```python
from build123d import *

# Parameters (mm, degrees)
EXTRUDE_1_DEPTH     = 10
CUT_EXTRUDE_1_DEPTH = 140.112364655
SKETCH_3_W          = 30
SKETCH_3_H          = 10
SKETCH_3_W_2        = 75
SKETCH_3_H_2        = 20
CUT_EXTRUDE_2_DEPTH = 140.112364655
SKETCH_4_W          = 25
SKETCH_4_H          = 10
EXTRUDE_2_DEPTH     = 4.5
CUT_EXTRUDE_3_DEPTH = 141.071410359


with BuildPart() as part:
    # 草圖1 → 填料-伸長1 (new body)
    with BuildSketch(Plane.XY):
        Polygon((136, -22.5), (136, -7.5), (130, -7.5), (130, 7.5), (136, 7.5), (136, 22.5), (-136, 22.5), (-136, 7.5), (-130, 7.5), (-130, -7.5), (-136, -7.5), (-136, -22.5), (-130, -22.5), (-130, -27.5), (130, -27.5), (130, -22.5), align=None)
        with BuildLine():
            Line((-31.35, -22.5), (-31.35, -2.5))
            ThreePointArc((-31.35, -2.5), (-30, -1.15), (-28.65, -2.5))
            Line((-28.65, -2.5), (-28.65, -22.5))
            ThreePointArc((-28.65, -22.5), (-30, -23.85), (-31.35, -22.5))
        make_face(mode=Mode.SUBTRACT)
        with BuildLine():
            Line((31.35, -22.5), (31.35, -2.5))
            ThreePointArc((31.35, -2.5), (30, -1.15), (28.65, -2.5))
            Line((28.65, -2.5), (28.65, -22.5))
            ThreePointArc((28.65, -22.5), (30, -23.85), (31.35, -22.5))
        make_face(mode=Mode.SUBTRACT)
    extrude(amount=EXTRUDE_1_DEPTH)

    # 草圖2 → 除料-伸長1 (cut, through all)
    with BuildSketch(Plane.XY.offset(10)):
        with BuildLine():
            Line((-92.5, 19.1), (-52.5, 19.1))
            ThreePointArc((-52.5, 19.1), (-49.4, 16), (-52.5, 12.9))
            Line((-52.5, 12.9), (-92.5, 12.9))
            ThreePointArc((-92.5, 12.9), (-95.6, 16), (-92.5, 19.1))
        make_face()
        with BuildLine():
            Line((-92.5, -15.9), (-52.5, -15.9))
            ThreePointArc((-52.5, -15.9), (-49.4, -19), (-52.5, -22.1))
            Line((-52.5, -22.1), (-92.5, -22.1))
            ThreePointArc((-92.5, -22.1), (-95.6, -19), (-92.5, -15.9))
        make_face()
        with BuildLine():
            Line((52.5, 19.1), (92.5, 19.1))
            ThreePointArc((92.5, 19.1), (95.6, 16), (92.5, 12.9))
            Line((92.5, 12.9), (52.5, 12.9))
            ThreePointArc((52.5, 12.9), (49.4, 16), (52.5, 19.1))
        make_face()
        with BuildLine():
            Line((52.5, -15.9), (92.5, -15.9))
            ThreePointArc((92.5, -15.9), (95.6, -19), (92.5, -22.1))
            Line((92.5, -22.1), (52.5, -22.1))
            ThreePointArc((52.5, -22.1), (49.4, -19), (52.5, -15.9))
        make_face()
    extrude(amount=-CUT_EXTRUDE_1_DEPTH, mode=Mode.SUBTRACT)

    # 草圖3 → 除料-伸長2 (cut, through all)
    with BuildSketch(Plane.XY.offset(10)):
        with Locations((0, -22.5)):
            Rectangle(SKETCH_3_W, SKETCH_3_H)
        with Locations((0, 12.5)):
            Rectangle(SKETCH_3_W_2, SKETCH_3_H_2)
    extrude(amount=-CUT_EXTRUDE_2_DEPTH, mode=Mode.SUBTRACT)

    # 草圖4 → 填料-伸長2 (add)
    with BuildSketch(Plane.XZ.offset(27.5)):
        with Locations((-27.5, 5)):
            Rectangle(SKETCH_4_W, SKETCH_4_H)
        with Locations((27.5, 5)):
            Rectangle(SKETCH_4_W, SKETCH_4_H)
    extrude(amount=EXTRUDE_2_DEPTH)

    # 草圖5 → 除料-伸長3 (cut, through all)
    with BuildSketch(Plane.XY.offset(10)):
        with BuildLine():
            Line((-107.1, 13.45), (-107.1, 1.35))
            ThreePointArc((-107.1, 1.35), (-104.55, -1.2), (-102, 1.35))
            Line((-102, 1.35), (-102, 13.45))
            ThreePointArc((-102, 13.45), (-104.55, 16), (-107.1, 13.45))
        make_face()
        with BuildLine():
            Line((107.1, 13.45), (107.1, 1.35))
            ThreePointArc((107.1, 1.35), (104.55, -1.2), (102, 1.35))
            Line((102, 1.35), (102, 13.45))
            ThreePointArc((102, 13.45), (104.55, 16), (107.1, 13.45))
        make_face()
    extrude(amount=-CUT_EXTRUDE_3_DEPTH, mode=Mode.SUBTRACT)


solid = part.part
```
Input: part model. Units: mm. Frame: model coordinates. A direction names the side the tool comes from. Coordinates: 2 decimals unless noted, no trailing zeros. Loops run counter-clockwise (first coordinate to the right, second up) from the corner with the lowest first, then second, coordinate; pieces in that order, holes last. Notation, with made-up numbers: (-22.75, 68) -> (-13.75, 68) arc R22 ccw to (-13.75, 84) -> close; hole circle Ø10 at (88, 67). An arc over 180 degrees is marked (long way). Use a Markdown table: item, result.
1) Pull-direction query (X, two-part tool) for faces 4 (the flat face through (-107.1, 7, 5)), 5 (the flat face through (-28, -32, 5)), 6 (the flat face through (136, -15, 5)); classes: released by +X, released by -X, zero draft, split by the parting line, or undercut.
Results found:
| item | result |
|---|---|
| face 4 | undercut |
| face 5 | zero draft |
| face 6 | released by +X |
2) Cut plane C-C (z = 4). Give the number of separate pieces and of enclosed holes in the cut face, then the cut area to 3 significant figures.
Results found:
| item | result |
|---|---|
| separate pieces | 1 |
| enclosed holes | 8 |
| area | 10,400 mm2 |
3) Access query for faces 1 (the flat face through (-133, -22.5, 5)), 2 (the flat face through (-133, -7.5, 5)), 3 (the flat face through (-1, 2.5, 5)). Directions: +Z, -Z, +X, -X, +Y, -Y. A direction counts if a zero-diameter tool reaches every point of the face in a straight line with its end or side. Return the directions, or none.
Results found:
| item | result |
|---|---|
| face 1 | +Z, -Z, -X, -Y |
| face 2 | +Z, -Z, -X |
| face 3 | +Z, -Z, +Y |
4) Cut plane A-A (x = -104.55). Return the cut outline in (y, z), then the cut area to 3 significant figures.
Results found:
| item | result |
|---|---|
| outline | (-27.5, 0) -> (-1.2, 0) -> (-1.2, 10) -> (-27.5, 10) -> close; (16, 0) -> (22.5, 0) -> (22.5, 10) -> (16, 10) -> close |
| area | 328 mm2 |
5) Contact query for flat-ended pins moving along their axis: pin 1 (1.5 mm diameter, centred on x = 83.5, y = 0.5, fed in from -Z); pin 2 (1.3 mm diameter, centred on y = -29.5, z = 3, fed in from +X); pin 3 (2.5 mm diameter, centred on y = -24, z = 4, fed in from +X); pin 4 (2 mm diameter, centred on y = -3.5, z = 4.5, fed in from -X). Output: stop coordinate, or through.
Results found:
| item | result |
|---|---|
| pin 1 | stops at z = 0 |
| pin 2 | stops at x = 40 |
| pin 3 | stops at x = 130 |
| pin 4 | stops at x = -130 |
6) Material intervals for line 1 along X through (y, z) = (4, 2.25); line 2 along Y through (x, z) = (54, 3); line 3 along Y through (x, z) = (30, 6), sorted ascending. Write a range as from..to.
Results found:
| item | result |
|---|---|
| line 1 | x = -130..-107.1, -102..-37.5, 37.5..102, 107.1..130 |
| line 2 | y = -27.5..-22.1, -15.9..12.9, 19.1..22.5 |
| line 3 | y = -32..-23.85, -1.15..2.5 |
7) Cut plane B-B (y = -12.5). Return the cut outline in (x, z), then the cut area to 3 significant figures.
Results found:
| item | result |
|---|---|
| outline | (-136, 0) -> (-31.35, 0) -> (-31.35, 10) -> (-136, 10) -> close; (-28.65, 0) -> (28.65, 0) -> (28.65, 10) -> (-28.65, 10) -> close; (31.35, 0) -> (136, 0) -> (136, 10) -> (31.35, 10) -> close |
| area | 2,670 mm2 |
